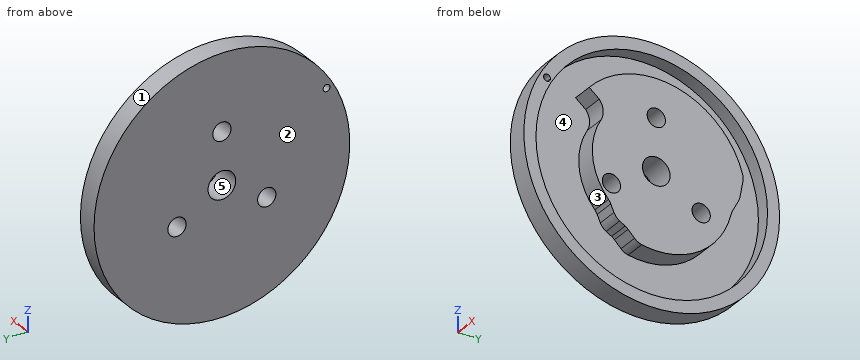
```python
from build123d import *

# Parameters (mm, degrees)
F0_R     = 37
F0_R_2   = 2.65
F0_R_3   = 4
F1_DEPTH = 8
F2_DEPTH = 2
F3_R     = 33.5
F4_DEPTH = 4


# Not quite as in the source:
# - a feature names something its author has since deleted; it is built from what else it names


with BuildPart() as f1:
    # F0 (on Right) → F1 (new body)
    with BuildSketch(Plane.YZ):
        Circle(F0_R)
        with BuildLine():
            ThreePointArc((-31.1769145362, 18), (-30.0520700874, 18.4659258263), (-29.3108891325, 17.5))
            ThreePointArc((-29.3108891325, 17.5), (-29.3449633062, 17.2411809549), (-29.4448637287, 17))
            ThreePointArc((-29.4448637287, 17), (-30.8108891325, 16.6339745962), (-31.1769145362, 18))
        make_face(mode=Mode.SUBTRACT)
        with BuildLine():
            ThreePointArc((-13.8307570654, -12.2865845131), (-18.4050260219, -1.8721690986), (-16.02146997, 9.25))
            ThreePointArc((-16.02146997, 9.25), (-15.3688742415, 12.1652999186), (-16.4950815942, 14.9323401783))
            Line((-16.4950815942, 14.9323401783), (-19.414607735, 17.2937273743))
            ThreePointArc((-19.414607735, 17.2937273743), (5.7943493018, 25.3461144195), (25.0003908736, 7.1400599553))
            ThreePointArc((25.0003908736, 7.1400599553), (25.1492760253, 6.2395359628), (25.0901387998, 5.3287050027))
            Line((25.0901387998, 5.3287050027), (24.230588756, 0.582974524))
            ThreePointArc((24.230588756, 0.582974524), (24.0836635039, 0.0139846058), (23.8549574473, -0.527337938))
            Line((23.8549574473, -0.527337938), (22.0020362781, -4.1457144451))
            ThreePointArc((22.0020362781, -4.1457144451), (21.8067059734, -4.5923170456), (21.6671490665, -5.0593627397))
            ThreePointArc((21.6671490665, -5.0593627397), (13.8291662627, -17.4303373599), (0, -22.25))
            ThreePointArc((0, -22.25), (-2.1048516517, -22.1502166925), (-4.1908242867, -21.851761755))
            ThreePointArc((-4.1908242867, -21.851761755), (-5.3214186468, -21.4518874672), (-6.2826715748, -20.7348547893))
            Line((-6.2826715748, -20.7348547893), (-8.1615589997, -18.8334098464))
            ThreePointArc((-8.1615589997, -18.8334098464), (-8.5623101549, -18.4787752012), (-9.0068129011, -18.1808078731))
            Line((-9.0068129011, -18.1808078731), (-10.5765097016, -17.2745430028))
            ThreePointArc((-10.5765097016, -17.2745430028), (-11.5533785454, -16.4821921034), (-12.2358922377, -15.4256563749))
            Line((-12.2358922377, -15.4256563749), (-13.1618084894, -13.3279283396))
            ThreePointArc((-13.1618084894, -13.3279283396), (-13.4557617662, -12.781226145), (-13.8307570654, -12.2865845131))
        make_face(mode=Mode.SUBTRACT)
        with BuildLine():
            ThreePointArc((-16.4950815942, 14.9323401783), (-15.3688742415, 12.1652999186), (-16.02146997, 9.25))
            ThreePointArc((-16.02146997, 9.25), (-18.4050260219, -1.8721690986), (-13.8307570654, -12.2865845131))
            ThreePointArc((-13.8307570654, -12.2865845131), (-13.4557617662, -12.781226145), (-13.1618084894, -13.3279283396))
            Line((-13.1618084894, -13.3279283396), (-12.2358922377, -15.4256563749))
            ThreePointArc((-12.2358922377, -15.4256563749), (-11.5533785454, -16.4821921034), (-10.5765097016, -17.2745430028))
            Line((-10.5765097016, -17.2745430028), (-9.0068129011, -18.1808078731))
            ThreePointArc((-9.0068129011, -18.1808078731), (-8.5623101549, -18.4787752012), (-8.1615589997, -18.8334098464))
            Line((-8.1615589997, -18.8334098464), (-6.2826715748, -20.7348547893))
            ThreePointArc((-6.2826715748, -20.7348547893), (-5.3214186468, -21.4518874672), (-4.1908242867, -21.851761755))
            ThreePointArc((-4.1908242867, -21.851761755), (-2.1048516517, -22.1502166925), (0, -22.25))
            ThreePointArc((0, -22.25), (13.8291662627, -17.4303373599), (21.6671490665, -5.0593627397))
            ThreePointArc((21.6671490665, -5.0593627397), (21.8067059734, -4.5923170456), (22.0020362781, -4.1457144451))
            Line((22.0020362781, -4.1457144451), (23.8549574473, -0.527337938))
            ThreePointArc((23.8549574473, -0.527337938), (24.0836635039, 0.0139846058), (24.230588756, 0.582974524))
            Line((24.230588756, 0.582974524), (25.0901387998, 5.3287050027))
            ThreePointArc((25.0901387998, 5.3287050027), (25.1492760253, 6.2395359628), (25.0003908736, 7.1400599553))
            ThreePointArc((25.0003908736, 7.1400599553), (5.7943493018, 25.3461144195), (-19.414607735, 17.2937273743))
            Line((-19.414607735, 17.2937273743), (-16.4950815942, 14.9323401783))
        make_face()
        with Locations((-12.9903810568, -7.5)):
            Circle(F0_R_2, mode=Mode.SUBTRACT)
        with Locations((12.9903810568, -7.5)):
            Circle(F0_R_2, mode=Mode.SUBTRACT)
        Circle(F0_R_3, mode=Mode.SUBTRACT)
        with Locations((0, 15)):
            Circle(F0_R_2, mode=Mode.SUBTRACT)
    extrude(amount=-F1_DEPTH)

    # F0 (on Right) → F2 (cut)
    with BuildSketch(Plane.YZ):
        Circle(F0_R)
        with BuildLine():
            ThreePointArc((-31.1769145362, 18), (-30.0520700874, 18.4659258263), (-29.3108891325, 17.5))
            ThreePointArc((-29.3108891325, 17.5), (-29.3449633062, 17.2411809549), (-29.4448637287, 17))
            ThreePointArc((-29.4448637287, 17), (-30.8108891325, 16.6339745962), (-31.1769145362, 18))
        make_face(mode=Mode.SUBTRACT)
        with BuildLine():
            ThreePointArc((-13.8307570654, -12.2865845131), (-18.4050260219, -1.8721690986), (-16.02146997, 9.25))
            ThreePointArc((-16.02146997, 9.25), (-15.3688742415, 12.1652999186), (-16.4950815942, 14.9323401783))
            Line((-16.4950815942, 14.9323401783), (-19.414607735, 17.2937273743))
            ThreePointArc((-19.414607735, 17.2937273743), (5.7943493018, 25.3461144195), (25.0003908736, 7.1400599553))
            ThreePointArc((25.0003908736, 7.1400599553), (25.1492760253, 6.2395359628), (25.0901387998, 5.3287050027))
            Line((25.0901387998, 5.3287050027), (24.230588756, 0.582974524))
            ThreePointArc((24.230588756, 0.582974524), (24.0836635039, 0.0139846058), (23.8549574473, -0.527337938))
            Line((23.8549574473, -0.527337938), (22.0020362781, -4.1457144451))
            ThreePointArc((22.0020362781, -4.1457144451), (21.8067059734, -4.5923170456), (21.6671490665, -5.0593627397))
            ThreePointArc((21.6671490665, -5.0593627397), (13.8291662627, -17.4303373599), (0, -22.25))
            ThreePointArc((0, -22.25), (-2.1048516517, -22.1502166925), (-4.1908242867, -21.851761755))
            ThreePointArc((-4.1908242867, -21.851761755), (-5.3214186468, -21.4518874672), (-6.2826715748, -20.7348547893))
            Line((-6.2826715748, -20.7348547893), (-8.1615589997, -18.8334098464))
            ThreePointArc((-8.1615589997, -18.8334098464), (-8.5623101549, -18.4787752012), (-9.0068129011, -18.1808078731))
            Line((-9.0068129011, -18.1808078731), (-10.5765097016, -17.2745430028))
            ThreePointArc((-10.5765097016, -17.2745430028), (-11.5533785454, -16.4821921034), (-12.2358922377, -15.4256563749))
            Line((-12.2358922377, -15.4256563749), (-13.1618084894, -13.3279283396))
            ThreePointArc((-13.1618084894, -13.3279283396), (-13.4557617662, -12.781226145), (-13.8307570654, -12.2865845131))
        make_face(mode=Mode.SUBTRACT)
    extrude(amount=-F2_DEPTH, mode=Mode.SUBTRACT)

    # F3 (on face) → F4 (cut)
    with BuildSketch(Plane.YZ.offset(-2)):
        Circle(F3_R)
        with BuildLine():
            ThreePointArc((-13.8307570654, -12.2865845131), (-18.4050260219, -1.8721690986), (-16.02146997, 9.25))
            ThreePointArc((-16.02146997, 9.25), (-15.3688742415, 12.1652999186), (-16.4950815942, 14.9323401783))
            Line((-16.4950815942, 14.9323401783), (-19.414607735, 17.2937273743))
            ThreePointArc((-19.414607735, 17.2937273743), (5.7943493018, 25.3461144195), (25.0003908736, 7.1400599553))
            ThreePointArc((25.0003908736, 7.1400599553), (25.1492760253, 6.2395359628), (25.0901387998, 5.3287050027))
            Line((25.0901387998, 5.3287050027), (24.230588756, 0.582974524))
            ThreePointArc((24.230588756, 0.582974524), (24.0836635039, 0.0139846058), (23.8549574473, -0.527337938))
            Line((23.8549574473, -0.527337938), (22.0020362781, -4.1457144451))
            ThreePointArc((22.0020362781, -4.1457144451), (21.8067059734, -4.5923170456), (21.6671490665, -5.0593627397))
            ThreePointArc((21.6671490665, -5.0593627397), (12.1182361804, -18.6604086739), (-4.1908242867, -21.851761755))
            ThreePointArc((-4.1908242867, -21.851761755), (-5.3214186468, -21.4518874672), (-6.2826715748, -20.7348547893))
            Line((-6.2826715748, -20.7348547893), (-8.1615589997, -18.8334098464))
            ThreePointArc((-8.1615589997, -18.8334098464), (-8.5623101549, -18.4787752012), (-9.0068129011, -18.1808078731))
            Line((-9.0068129011, -18.1808078731), (-10.5765097016, -17.2745430028))
            ThreePointArc((-10.5765097016, -17.2745430028), (-11.5533785454, -16.4821921034), (-12.2358922377, -15.4256563749))
            Line((-12.2358922377, -15.4256563749), (-13.1618084894, -13.3279283396))
            ThreePointArc((-13.1618084894, -13.3279283396), (-13.4557617662, -12.781226145), (-13.8307570654, -12.2865845131))
        make_face(mode=Mode.SUBTRACT)
    extrude(amount=-F4_DEPTH, mode=Mode.SUBTRACT)


solid = f1.part
```
The listing builds one solid part. Answer for the finished solid, in the listing's coordinates (mm). Face numbers are marked on the shaded views. A direction names the side the tool comes from. Give positions to 0.01 mm unless a question says otherwise; leave off trailing zeros. Order: outer loops, then holes, each group sorted by start corner. A loop starts at its lowest first (then second) coordinate and runs counter-clockwise, first axis right, second up. Notation, with made-up numbers: (34, 24) -> (69, 24) arc R5 cw to (69, 31) -> close; hole circle Ø7 at (50.25, 36.25). An arc over 180 degrees is marked (long way). Answer as a JSON object with one key per item and string values. Group by question number.
Item 1: The part is cut by section B-B on z = -7.5. Write down the section's boundary in (x, y).
Item 2: The part is cut by section C-C on y = -17.5. Write down the section's boundary in (x, z).
Item 3: The part is cut by section A-A on x = -3.5. Write down the section's boundary in (y, z), and give its area (3 significant figures).
Item 4: Determine the mould class of the marked faces 1, 2 and 3 for opening direction Z: pulls with the +Z half, pulls with the -Z half, needs draft (parallel to the pull), parting line crosses it, or undercut.
Item 5: Consider L1, parallel to Z at x = -4, y = 0; L2, parallel to Z at x = -3, y = 12; L3, parallel to Y at x = -4, z = 11. Determine where each line is inside the solid, lowest interval first. Write a range as from..to.
Item 6: A tool of negligible diameter and unlimited length cuts with its end or side. For the marked faces 4 and 5, from which of +Z, -Z, +X, -X, +Y, -Y can it reach the whole face along a straight path? Write none if from no direction.
Item 7: The part is cut by section D-D on z = 19.5. Write down the section's boundary in (x, y), and give its area (3 significant figures).
Item 8: Flat-ended cylindrical pins translate along their axes: pin 1 (1 mm diameter, centred on x = -2, y = -5, fed in from +Z); pin 2 (2 mm diameter, centred on x = -5.5, y = -16, fed in from +Z); pin 3 (3 mm diameter, centred on y = -12.99, z = -7.5, fed in from -X); pin 4 (1 mm diameter, centred on x = -4, y = -4, fed in from -Z). Find the tip coordinate at first contact, or state that the pin passes through.
Result set:
{
 "1": {"outline": "(-8, -36.23) -> (-2, -36.23) -> (-2, -32.65) -> (-6, -32.65) -> (-6, -16.91) -> (0, -16.91) -> (0, -15.64) -> (-8, -15.64) -> close; (-8, -10.34) -> (0, -10.34) -> (0, 10.34) -> (-8, 10.34) -> close; (-8, 15.64) -> (0, 15.64) -> (0, 20.95) -> (-6, 20.95) -> (-6, 32.65) -> (-2, 32.65) -> (-2, 36.23) -> (-8, 36.23) -> close"},
 "2": {"outline": "(-8, -32.6) -> (-2, -32.6) -> (-2, -28.57) -> (-6, -28.57) -> (-6, -6) -> (0, -6) -> (0, 6) -> (-6, 6) -> (-6, 15.75) -> (0, 15.75) -> (0, 19.23) -> (-6, 19.23) -> (-6, 28.57) -> (-2, 28.57) -> (-2, 32.6) -> (-8, 32.6) -> close"},
 "3": {"outline": "circle Ø74 at (0, 0); (-19.41, 17.29) -> (-16.5, 14.93) arc R5 cw to (-16.02, 9.25) arc R18.5 ccw to (-13.83, -12.29) arc R4 cw to (-13.16, -13.33) -> (-12.24, -15.43) arc R4 ccw to (-10.58, -17.27) -> (-9.01, -18.18) arc R4 cw to (-8.16, -18.83) -> (-6.28, -20.73) arc R4 ccw to (-4.19, -21.85) arc R22.25 ccw to (21.67, -5.06) arc R4 cw to (22, -4.15) -> (23.85, -0.53) arc R4 ccw to (24.23, 0.58) -> (25.09, 5.33) arc R4 ccw to (25, 7.14) arc R26 ccw to start; hole circle Ø67 at (0, 0); hole circle Ø2 at (-30.31, 17.5); hole circle Ø5.3 at (-12.99, -7.5); hole circle Ø8 at (0, 0); hole circle Ø5.3 at (0, 15); hole circle Ø5.3 at (12.99, -7.5)", "area": "2,290 mm²"},
 "4": {"face 1": "parting line crosses it", "face 2": "needs draft", "face 3": "undercut"},
 "5": {"L1": "-37..-33.5, -22.25..-4, 4..12.35, 17.65..26, 33.5..37", "L2": "-35..-31.28, -18.74..-9.96, -5.04..23.07, 31.28..35", "L3": "-35.33..-31.64, -15.41..23.56, 31.64..35.33"},
 "6": {"face 4": "+X", "face 5": "+X, -X"},
 "7": {"outline": "(-8, -31.44) -> (-2, -31.44) -> (-2, -27.24) -> (-6, -27.24) -> (-6, -17.2) -> (0, -17.2) -> (0, 17.2) -> (-6, 17.2) -> (-6, 27.24) -> (-2, 27.24) -> (-2, 31.44) -> (-8, 31.44) -> close", "area": "366 mm²"},
 "8": {"pin 1": "z = 36.73", "pin 2": "z = 33.82", "pin 3": "through", "pin 4": "z = -36.83"}
}
